Geometry: final body of the model. Coordinates: model frame, mm. Give positions to 0.01 mm unless a question says otherwise; leave off trailing zeros. Write each loop counter-clockwise with the first axis right and the second up, starting at its lowest first coordinate (ties: lowest second). Pieces come first, ordered by that corner, then holes. Notation, with made-up numbers: (-22.75, 59) -> (-3.75, 59) arc R31 ccw to (-3.75, 96) -> close; hole circle Ø1 at (10.5, 25). An arc over 180 degrees is marked (long way). Answer as a JSON object with one key per item and string values.
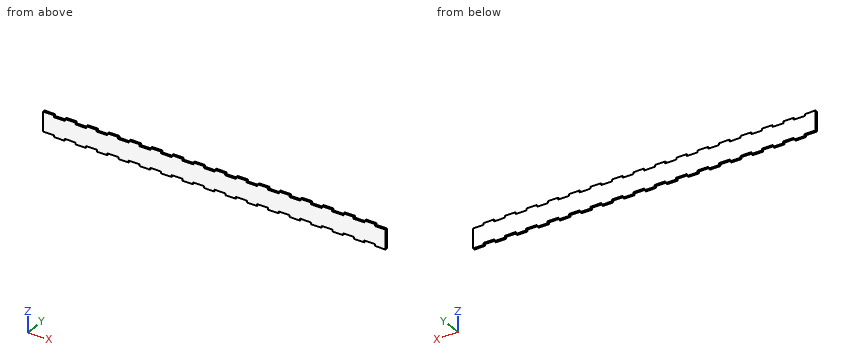
from build123d import *

# Parameters (mm, degrees)
SKETCH1_W           = 640
SKETCH1_H           = 40.4
BOSS_EXTRUDE1_DEPTH = 4
SKETCH2_W           = 20.6
SKETCH2_H           = 3.5
CUT_EXTRUDE1_DEPTH  = 4
LPATTERN1_COUNT     = 17
LPATTERN1_PITCH     = 40


with BuildPart() as part:
    # Sketch1 → Boss-Extrude1 (new body)
    with BuildSketch(Plane(origin=(0, 0, 0), x_dir=(1, 0, 0), z_dir=(0, 1, 0))):
        Rectangle(SKETCH1_W, SKETCH1_H)
    extrude(amount=BOSS_EXTRUDE1_DEPTH)

    # Sketch2 → Cut-Extrude1 (cut)
    with BuildSketch(Plane(origin=(0, 4, 0), x_dir=(1, 0, 0), z_dir=(0, 1, 0))):
        with Locations((-309.7, 18.45)):
            Rectangle(SKETCH2_W, SKETCH2_H)
        with Locations((-289.4, -18.45)):
            Rectangle(SKETCH2_W, SKETCH2_H)
    cut_extrude1 = extrude(amount=-CUT_EXTRUDE1_DEPTH, mode=Mode.SUBTRACT)

    # LPattern1: Cut-Extrude1 ×17
    with Locations(*[(i * LPATTERN1_PITCH, 0, 0) for i in range(1, LPATTERN1_COUNT)]):
        add(cut_extrude1, mode=Mode.SUBTRACT)


solid = part.part
Q1. First-contact query: P1, Ø2, axis at x = 206.5, y = 1.5, coming from the -Z side; P2, Ø2, axis at x = 73.5, y = 1.5, coming from the +Z side; P3, Ø1, axis at y = 2, z = 18.5, coming from the +X side. Flat tips, straight axial feed; report the tip coordinate or a pass-through.
Values:
{"P1": "z = -16.7", "P2": "z = 16.7", "P3": "x = 300.3"}
Q2. Material intervals for L1, parallel to Z at x = 91, y = 2.4; L2, parallel to Z at x = -239.5, y = 1.05, sorted ascending. Write a range as from..to.
Values:
{"L1": "-16.7..20.2", "L2": "-16.7..16.7"}
Q3. Cut plane A-A (x = 110). Return the cut outline in (y, z), and give its area (3 significant figures).
Values:
{"outline": "(0, -20.2) -> (4, -20.2) -> (4, 16.7) -> (0, 16.7) -> close", "area": "148 mm²"}
